Check sheet for the modelled part. Datum: model origin and axes. Units: mm. Face numbers are marked on the shaded views. A direction names the side the tool comes from. Coordinates: 2 decimals unless noted, no trailing zeros. Loops run counter-clockwise (first coordinate to the right, second up) from the corner with the lowest first, then second, coordinate; pieces in that order, holes last.
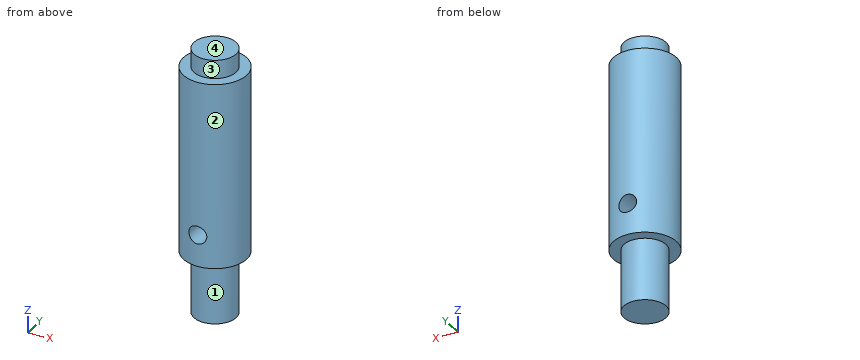
Autodesk Inventor part; units mm, degrees
ref_plane "作業平面1" through (0, 6, -21.175) normal (0, 1, 0) x (-1, 0, 0)
ref_plane "YZ Plane" through (0, 0, 0) normal (1, 0, 0) x (0, 1, 0)
ref_plane "XY Plane" through (0, 0, 0) normal (0, 0, 1) x (1, 0, 0)
sketch "スケッチ2" plane through (0, 0, 0) normal (1, 0, 0) x (0, 1, 0)
  line L0 (0, 0) -> (6, 0)
  line L1 (6, 0) -> (6, -50.65)
  line L2 (6, -50.65) -> (0, -50.65)
  line L3 (0, -50.65) -> (0, 0)
  line L4 (6, 0) -> (4, 0)
  line L5 (4, 0) -> (4, -3.5)
  line L6 (4, -3.5) -> (6, -3.5)
  line L7 (6, -3.5) -> (6, 0)
  line L8 (6, -50.65) -> (4, -50.65)
  line L9 (4, -50.65) -> (4, -38.85)
  line L10 (4, -38.85) -> (6, -38.85)
  line L11 (6, -38.85) -> (6, -50.65)
  dimension "d3" = 6
  dimension "d4" = 50.65
  dimension "d5" = 2
  dimension "d6" = 3.5
  dimension "d7" = 2
  dimension "d8" = 11.8
revolve "回転1" add sketch "スケッチ2" angle 360 about axis through (0, 0, -50.65) along (0, 0, 1) contours L0 L5 L6 L1 L10 L9 L2 L3
ref_plane "作業平面1" through (0, 6, -21.175) normal (0, 1, 0) x (-1, 0, 0)
sketch "スケッチ3" plane through (0, 6, -21.175) normal (0, 1, 0) x (-1, 0, 0)
  line L0 (4, 21.175) -> (-4, 21.175)
  point P0 (0, 21.175)
  point P1 (0, -11.675)
  dimension "d10" = 32.85
hole "穴1" at (0, 6, -32.85) direction (0, -1, 0) diameter 3.4 end through all
properties part number "install-encoder-v1-Shaft-E-Shaft" material "アルミニウム 6061"
1) Section check D-D on y = 3.5. Enter the section's corners in (x, z), plus the area to 3 significant figures.
Answer sheet:
outline: (-4.87, -38.85) - (-1.94, -38.85) - (-1.94, -50.65) - (1.94, -50.65) - (1.94, -38.85) - (4.87, -38.85) - (4.87, -3.5) - (1.94, -3.5) - (1.94, 0) - (-1.94, 0) - (-1.94, -3.5) - (-4.87, -3.5) - close; hole circle Ø3.4 at (0, -32.85)
area: 395 mm2
2) Set-up check for the marked faces 1 and 2: record each of +Z, -Z, +X, -X, +Y, -Y from which the full face is reachable in a straight line by a thin tool's end or side.
Answer sheet:
face 1: -Z
face 2: +Z, -Z
3) Section check C-C on z = -32.85. Enter the section's corners in (x, y), plus the area to 4 significant figures.
Answer sheet:
outline: (-1.7, -5.75) - (-1.7, 5.75) arc R6 ccw to start; (1.7, -5.75) arc R6 ccw to (1.7, 5.75) - close
area: 72.85 mm2
4) Depth check by flat-ended pin: pin 1 (1.5 mm diameter, centred on y = 3.5, z = -25.5, fed in from +X); pin 2 (1 mm diameter, centred on x = -1.5, z = -31, fed in from +Y); pin 3 (4 mm diameter, centred on x = 2.5, z = -33.5, fed in from -Y). Enter the tip coordinate at first touch or a pass-through.
Answer sheet:
pin 1: stops at x = 5.33
pin 2: stops at y = 5.92
pin 3: stops at y = -5.96
5) Section check A-A on x = 0. Enter the section's corners in (y, z).
Answer sheet:
outline: (-6, -38.85) - (-4, -38.85) - (-4, -50.65) - (4, -50.65) - (4, -38.85) - (6, -38.85) - (6, -34.55) - (-6, -34.55) - close; (-6, -31.15) - (6, -31.15) - (6, -3.5) - (4, -3.5) - (4, 0) - (-4, 0) - (-4, -3.5) - (-6, -3.5) - close
6) Section check B-B on y = 0. Enter the section's corners in (x, z).
Answer sheet:
outline: (-6, -38.85) - (-4, -38.85) - (-4, -50.65) - (4, -50.65) - (4, -38.85) - (6, -38.85) - (6, -3.5) - (4, -3.5) - (4, 0) - (-4, 0) - (-4, -3.5) - (-6, -3.5) - close; hole circle Ø3.4 at (0, -32.85)
7) Mould release check, pull along X, two halves, no side actions. Record for the marked faces 3 and 4: +X half, -X half, draft (parallel to the pull), parting line (faces both ways), or undercut.
Answer sheet:
face 3: parting line
face 4: draft
8) Scan lines: line 1 (Z direction, x = 0, y = 3); line 2 (Z direction, x = -4, y = 4.25); line 3 (X direction, y = 2, z = -32.85). Record each from-to range of solid material in increasing order.
Answer sheet:
line 1: z = -50.65 to -34.55, -31.15 to 0
line 2: z = -38.85 to -3.5
line 3: x = -5.66 to -1.7, 1.7 to 5.66
